Check sheet for the modelled part. Datum: model origin and axes. Units: mm. A direction names the side the tool comes from. Round coordinates to 2 decimals unless told otherwise and drop trailing zeros. Write each loop counter-clockwise with the first axis right and the second up, starting at its lowest first coordinate (ties: lowest second). Pieces come first, ordered by that corner, then holes.
Item 1: Cross-section at C-C on y = 27.5. Enter the section's corners in (x, z).
Item 2: Cross-section at A-A on z = -63.5. Enter the section's corners in (x, y), plus the area to 3 significant figures.
Item 3: Material ranges on line 1 (X direction, y = 3.8, z = -6.5); line 2 (X direction, y = 94, z = -41.5); line 3 (Z direction, x = -44, y = 3), recorded low to high.
Item 4: Cross-section at B-B on x = -44.5. Enter the section's corners in (y, z), plus the area to 3 significant figures.
Item 5: Release check for a two-part mould opening along Z. For faces 1 (the flat face through (-47.5, 56, -34)), 2 (the flat face through (-25, 52, -70)), 3 (the flat face through (-50, 52, -35)) record: +Z half, -Z half, draft (parallel to the pull), parting line (faces both ways), or undercut.
Item 6: Go/stop test with flat-tipped pins: pin 1 Ø1.8 at (x, z) = (-5.5, -63.5) entering from -Y; pin 2 Ø3 at (x, z) = (-18, -1.5) entering from +Y; pin 3 Ø4 at (x, y) = (-36.5, 89) entering from +Z. Record where each tip stops, or that it passes through.
Item 7: Cross-section at D-D on z = -19.5. Enter the section's corners in (x, y).
Item 8: Tool access check on faces 4 (the flat face through (-25, 75, -2)), 5 (the cylindrical face through (-43.17, 2.46, -62.81)), 6 (the flat face through (-25, 40, -3.5)). Record the directions out of +Z, -Z, +X, -X, +Y, -Y that give a thin tool (end or side, any length) a straight path to the whole face; none if there is none.
Autodesk Inventor part; units mm, degrees
ref_plane "YZ Plane" through (0, 0, 0) normal (1, 0, 0) x (0, 1, 0)
ref_plane "XZ Plane" through (0, 0, 0) normal (0, 1, 0) x (-1, 0, 0)
ref_plane "XY Plane" through (0, 0, 0) normal (0, 0, 1) x (1, 0, 0)
sketch "Sketch1" plane through (0, 0, 0) normal (0, 1, 0) x (-1, 0, 0)
  line L0 (0, 0) -> (50, 0)
  line L1 (50, 0) -> (50, -70)
  line L2 (50, -70) -> (0, -70)
  line L3 (0, -70) -> (0, 0)
  dimension "d0" = 50
  dimension "d1" = 70
extrude "Extrusion1" add sketch "Sketch1" along normal blind 5
sketch "Sketch2" plane through (0, 5, 0) normal (0, 1, 0) x (1, 0, 0)
  line L0 (0, 0) -> (-50, 0)
  line L1 (-50, 70) -> (0, 70)
  line L2 (-2.5, 66.5) -> (-47.5, 66.5)
  line L3 (-47.5, 66.5) -> (-47.5, 3.5)
  line L4 (-47.5, 3.5) -> (-2.5, 3.5)
  line L5 (-2.5, 3.5) -> (-2.5, 66.5)
  line L6 (0, 0) -> (0, 70)
  line L7 (-50, 70) -> (-50, 0)
  line L8 (0, 70) -> (-50, 70)
  line L9 (-50, 0) -> (0, 0)
  line L10 (0, 0) -> (0, 70)
  line L11 (0, 70) -> (-50, 70)
  line L12 (-50, 70) -> (-50, 0)
  dimension "d22" = 63
  dimension "d24" = 45
  dimension "d25" = 2.5
  dimension "d27" = 3.5
  dimension "d28" = 50
extrude "Extrusion2" add sketch "Sketch2" along normal blind 100
sketch "Sketch3" plane through (0, 5, 0) normal (0, 1, 0) x (1, 0, 0)
  point P0 (0, 0)
sketch "Sketch5" plane through (0, 5, 0) normal (0, 1, 0) x (1, 0, 0)
  line L0 (-47.5, 3.5) -> (-47.5, 66.5)
  line L1 (-2.5, 3.5) -> (-47.5, 3.5)
  line L2 (-2.5, 66.5) -> (-2.5, 3.5)
  line L3 (-47.5, 66.5) -> (-2.5, 66.5)
  point P0 (0, 0)
  point P1 (-44.5, 6.5)
  point P2 (-44.5, 63.5)
  point P3 (-5.5, 63.5)
  point P4 (-5.5, 6.5)
  dimension "d36" = 3
  dimension "d37" = 3
  dimension "d38" = 3
  dimension "d39" = 3
  dimension "d40" = 3
  dimension "d41" = 3
  dimension "d42" = 3
  dimension "d43" = 3
hole "Hole2" at (-44.5, 5, -6.5) at (-5.5, 5, -6.5) at (-5.5, 5, -63.5) at (-44.5, 5, -63.5) direction (0, -1, 0) diameter 3 end through all
sketch "Sketch6" plane through (0, 105, 0) normal (0, 1, 0) x (1, 0, 0)
  line L0 (-50, 0) -> (0, 0)
  line L1 (-2.5, 3.5) -> (-47.5, 3.5)
  line L2 (-47.5, 3.5) -> (-47.5, 0)
  line L3 (-47.5, 0) -> (-2.5, 0)
  line L4 (-2.5, 0) -> (-2.5, 3.5)
  point P0 (-2.5, 0)
  dimension "d44" = 45
extrude "Extrusion3" cut sketch "Sketch6" against normal blind 30
properties part number "poerbankhållare_3DPrint"
Response values:
1. outline: (-50, -70) - (0, -70) - (0, 0) - (-50, 0) - close; hole (-47.5, -66.5) - (-2.5, -66.5) - (-2.5, -3.5) - (-47.5, -3.5) - close
2. outline: (-50, 0) - (-46, 0) - (-46, 5) - (-47.5, 5) - (-47.5, 105) - (-50, 105) - close; (-43, 0) - (-7, 0) - (-7, 5) - (-43, 5) - close; (-4, 0) - (0, 0) - (0, 105) - (-2.5, 105) - (-2.5, 5) - (-4, 5) - close
2. area: 720 mm2
3. line 1: x = -50 to -46, -43 to -7, -4 to 0
3. line 2: x = -50 to -47.5, -2.5 to 0
3. line 3: z = -70 to -64.91, -62.09 to -7.91, -5.09 to 0
4. outline: (0, -70) - (105, -70) - (105, -66.5) - (5, -66.5) - (5, -65) - (0, -65) - close; (0, -62) - (5, -62) - (5, -8) - (0, -8) - close; (0, -5) - (5, -5) - (5, -3.5) - (75, -3.5) - (75, 0) - (0, 0) - close
4. area: 915 mm2
5. face 1: undercut
5. face 2: -Z half
5. face 3: draft
6. pin 1: passes through
6. pin 2: stops at y = 75
6. pin 3: stops at z = -66.5
7. outline: (-50, 0) - (0, 0) - (0, 105) - (-2.5, 105) - (-2.5, 5) - (-47.5, 5) - (-47.5, 105) - (-50, 105) - close
8. face 4: +Z, +Y
8. face 5: +Y, -Y
8. face 6: +Y
